Design review of the part shown in the three views and the two pictorial views. Dimensions are in mm from the part's minimum x, y and z. A direction names the side the tool comes from. Give positions to 0.01 mm unless a question says otherwise; leave off trailing zeros. Order: outer loops, then holes, each group sorted by start corner. A loop starts at its lowest first (then second) coordinate and runs counter-clockwise, first axis right, second up. Notation, with made-up numbers: (8.5, 57) - (18.5, 57) arc R18 cw to (18.5, 69) - close; hole circle Ø6 at (1.5, -34.5). An arc over 180 degrees is marked (long way). Put each result on its own line as item: value.
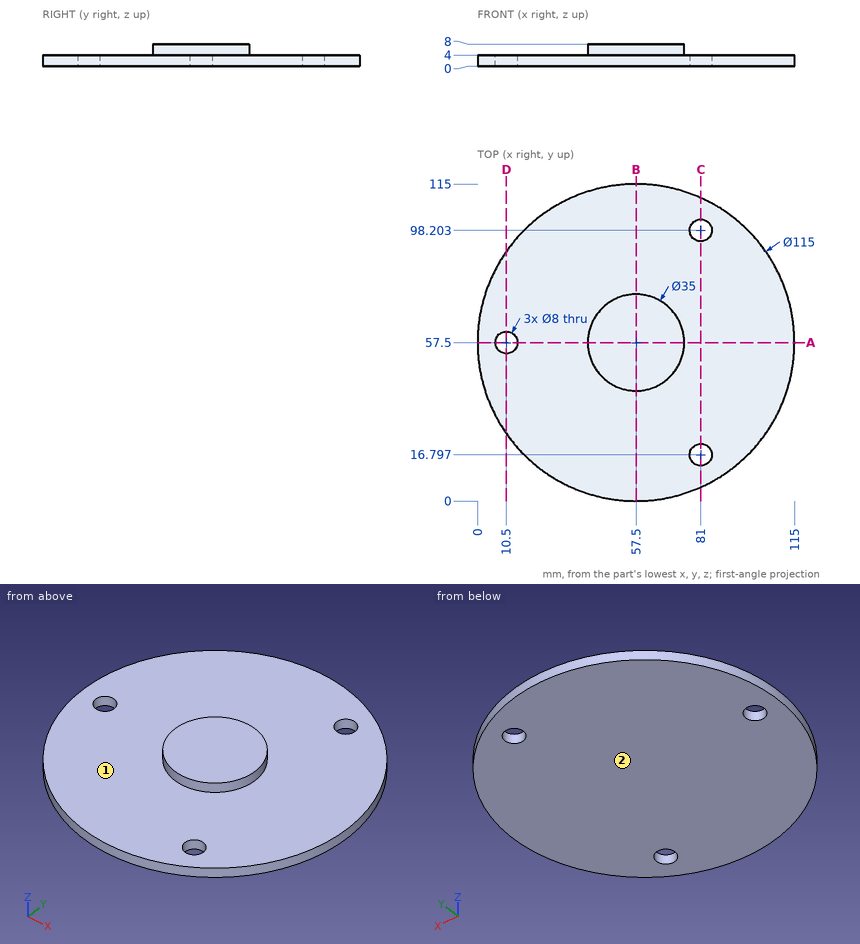
(1) Clearance check with flat-ended pins moving along their axes: pin 1 Ø1.5 at (x, y) = (102, 73) entering from +Z; pin 2 Ø6 at (x, y) = (17, 15) entering from -Z. State where each tip first meets the part, or that it passes through.
The answers:
pin 1: z = 4
pin 2: z = 0
(2) Wall thickness on L1, parallel to Y at x = 81, z = 2.65; L2, parallel to Z at x = 71, y = 6.5; L3, parallel to Y at x = 58, z = 5: over which ranges is each line inside the solid? List them lowest first.
The answers:
L1: 5.02 to 12.8, 20.8 to 94.2, 102.2 to 109.98
L2: 0 to 4
L3: 40.01 to 74.99
(3) Take a section at C-C, the plane x = 81. Write out the cut boundary in (y, z).
The answers:
outline: (5.02, 0) - (12.8, 0) - (12.8, 4) - (5.02, 4) - close; (20.8, 0) - (94.2, 0) - (94.2, 4) - (20.8, 4) - close; (102.2, 0) - (109.98, 0) - (109.98, 4) - (102.2, 4) - close
(4) Take a section at D-D, the plane x = 10.5. Write out the cut boundary in (y, z) (1 decimal), then the cut area to 3 significant figures.
The answers:
outline: (24.4, 0) - (53.5, 0) - (53.5, 4) - (24.4, 4) - close; (61.5, 0) - (90.6, 0) - (90.6, 4) - (61.5, 4) - close
area: 233 mm^2
(5) For the marked faces 1 and 2, list the 3-axis set-ups (+Z, -Z, +X, -X, +Y, -Y) from which the entire face can be reached by the end or side of a thin tool; tool diameter is ignored.
The answers:
face 1: +Z
face 2: -Z, +X, -X, +Y, -Y
(6) Take a section at B-B, the plane x = 57.5. Write out the cut boundary in (y, z), then the cut area to 3 significant figures.
The answers:
outline: (0, 0) - (115, 0) - (115, 4) - (75, 4) - (75, 8) - (40, 8) - (40, 4) - (0, 4) - close
area: 600 mm^2
(7) Take a section at A-A, the plane y = 57.5. Write out the cut boundary in (x, z), then the cut area to 3 significant figures.
The answers:
outline: (0, 0) - (6.5, 0) - (6.5, 4) - (0, 4) - close; (14.5, 0) - (115, 0) - (115, 4) - (75, 4) - (75, 8) - (40, 8) - (40, 4) - (14.5, 4) - close
area: 568 mm^2
